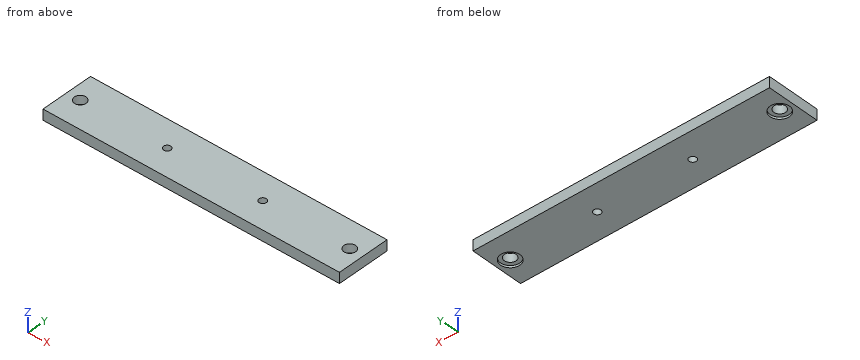
Autodesk Fusion 360 part; units mm, degrees
sketch "Sketch1" plane through (0, 0, 0) normal (0, 0, 1) x (1, 0, 0)
  line L0 (0, 0) -> (139.7, 0)
  line L1 (139.7, 0) -> (139.7, 25)
  line L2 (139.7, 25) -> (0, 25)
  line L3 (0, 25) -> (0, 0)
  dimension "d1" = 139.7
  dimension "d2" = 25
extrude "Extrude1" add sketch "Sketch1" along normal blind 5
sketch "Sketch2" plane through (0, 0, 0) normal (0, 0, 1) x (1, 0, 0)
  point P0 (6.35, 12.5)
  point P1 (133.35, 12.5)
hole "Hole1" at (6.35, 12.5, 0) at (133.35, 12.5, 0) direction (0, 0, 1) diameter 5.5 depth 13 tip angle 118 counterbore diameter 9.1 counterbore depth 1
sketch "Sketch4" plane through (0, 0, 0) normal (0, 0, -1) x (1, 0, 0)
  circle A0 centre (6.35, -12.5) radius 4.55
  circle A1 centre (133.35, -12.5) radius 4.55
  line L0 (0, 0) -> (0, -25)
  line L1 (0, -25) -> (139.7, -25)
  line L2 (139.7, -25) -> (139.7, 0)
  line L3 (139.7, 0) -> (0, 0)
  point P0 (47.35, -12.5)
  point P1 (92.35, -12.5)
hole "Hole3" at (92.35, 12.5, 0) at (47.35, 12.5, 0) direction (0, 0, 1) diameter 3.4 depth 13 tip angle 118
For this review, take the finished solid that the model builds, in its own axes (mm). Give positions to 0.01 mm unless a question says otherwise; leave off trailing zeros. Order: outer loops, then holes, each group sorted by start corner. A loop starts at its lowest first (then second) coordinate and runs counter-clockwise, first axis right, second up. Notation, with made-up numbers: (60.25, -20.75) -> (95.25, -20.75) arc R22 ccw to (95.25, -3.75) -> close; hole circle Ø9 at (22, -40). An arc over 180 degrees is marked (long way). Write item = value, one per line.
1) We need section C-C, the plane z = 3.9. Give the boundary of the cut face in (x, y), and give its area (3 significant figures).
Findings:
outline = (0, 0) -> (139.7, 0) -> (139.7, 25) -> (0, 25) -> close; hole circle Ø5.5 at (6.35, 12.5); hole circle Ø3.4 at (47.35, 12.5); hole circle Ø3.4 at (92.35, 12.5); hole circle Ø5.5 at (133.35, 12.5)
area = 3,430 mm^2
2) We need section A-A, the plane x = 47.35. Give the boundary of the cut face in (y, z).
Findings:
outline = (0, 0) -> (10.8, 0) -> (10.8, 5) -> (0, 5) -> close; (14.2, 0) -> (25, 0) -> (25, 5) -> (14.2, 5) -> close
3) Insertion check: pin 1 (5 mm diameter, centred on x = 6.35, y = 12.5, fed in from -Z); pin 2 (4.5 mm diameter, centred on x = 4.5, y = 11.5, fed in from -Z). Each pin has a flat end and moves straight along its axis. Give the tip position at first contact, or say it passes through.
Findings:
pin_1 = through
pin_2 = 1
4) We need section B-B, the plane y = 12.5. Give the boundary of the cut face in (x, z).
Findings:
outline = (0, 0) -> (1.8, 0) -> (1.8, 1) -> (3.6, 1) -> (3.6, 5) -> (0, 5) -> close; (9.1, 1) -> (10.9, 1) -> (10.9, 0) -> (45.65, 0) -> (45.65, 5) -> (9.1, 5) -> close; (49.05, 0) -> (90.65, 0) -> (90.65, 5) -> (49.05, 5) -> close; (94.05, 0) -> (128.8, 0) -> (128.8, 1) -> (130.6, 1) -> (130.6, 5) -> (94.05, 5) -> close; (136.1, 1) -> (137.9, 1) -> (137.9, 0) -> (139.7, 0) -> (139.7, 5) -> (136.1, 5) -> close
5) We need section D-D, the plane x = 6.35. Give the boundary of the cut face in (y, z), and give its area (3 significant figures).
Findings:
outline = (0, 0) -> (7.95, 0) -> (7.95, 1) -> (9.75, 1) -> (9.75, 5) -> (0, 5) -> close; (15.25, 1) -> (17.05, 1) -> (17.05, 0) -> (25, 0) -> (25, 5) -> (15.25, 5) -> close
area = 93.9 mm^2
6) To check wall thickness, follow L1, parallel to X at y = 12.5, z = 3.3; L2, parallel to Y at x = 133.35, z = 3.5; L3, parallel to X at y = 12.5, z = 0.4. State the ranges of each line that lie inside material, in increasing order. Write a range as from..to.
Findings:
L1 = 0..3.6, 9.1..45.65, 49.05..90.65, 94.05..130.6, 136.1..139.7
L2 = 0..9.75, 15.25..25
L3 = 0..1.8, 10.9..45.65, 49.05..90.65, 94.05..128.8, 137.9..139.7
